Job drawing, mm, ordinate dimensions from the low corner. One solid piece. A direction names the side the tool comes from. Give positions to 0.01 mm unless a question says otherwise; leave off trailing zeros. Order: outer loops, then holes, each group sorted by start corner. A loop starts at its lowest first (then second) coordinate and runs counter-clockwise, first axis right, second up.
Item 1: Band-saw the part on C-C on z = 4.25. Give the cut face in (x, y).
Item 2: Band-saw the part on A-A on x = 15. Give the cut face in (y, z).
Item 3: Which spindle directions (+Z, -Z, +X, -X, +Y, -Y) get a long thin tool onto all of the face, cutting with end or side? Do the marked faces 1 and 2. Say none if no direction does.
Item 4: Band-saw the part on D-D on z = 14.25. Give the cut face in (x, y).
Item 5: Flat gauge pins, fed straight in: P1, Ø3, axis at y = 25, z = 2.5, coming from the -X side; P2, Ø1.6, axis at x = 15, y = 25, coming from the -Z side; P3, Ø2.5, axis at x = 23.66, y = 10, coming from the +Z side. Where does each tip first touch, or does it go through?
Item 6: Band-saw the part on B-B on z = 8.5. Give the cut face in (x, y).
Item 7: Wall check: L1, parallel to Y at x = 15, z = 3.75; L2, parallel to Y at x = 7, z = 2.5; L3, parallel to Z at x = 6, y = 22.5. Give the ranges that are in metal, low to high.
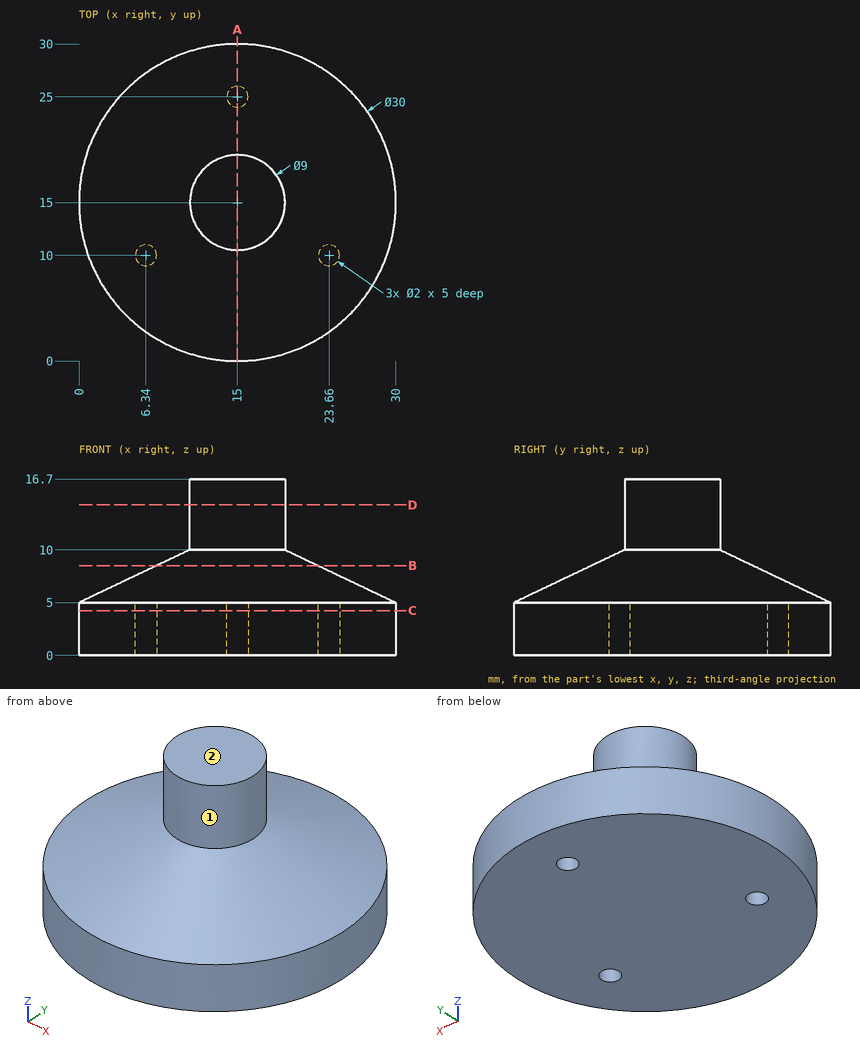
The answers:
1. outline: circle Ø30 at (15, 15); hole circle Ø2 at (6.34, 10); hole circle Ø2 at (15, 25); hole circle Ø2 at (23.66, 10)
2. outline: (0, 0) - (24, 0) - (24, 5) - (26, 5) - (26, 0) - (30, 0) - (30, 5) - (19.5, 10) - (19.5, 16.7) - (10.5, 16.7) - (10.5, 10) - (0, 5) - close
3. face 1: +Z
3. face 2: +Z, +X, -X, +Y, -Y
4. outline: circle Ø9 at (15, 15)
5. P1: stops at x = 2.64
5. P2: stops at z = 5
5. P3: stops at z = 7.98
6. outline: circle Ø15.3 at (15, 15)
7. L1: y = 0 to 24, 26 to 30
7. L2: y = 2.31 to 9.25, 10.75 to 27.69
7. L3: z = 0 to 6.56
